For this review, use the dimensioned drawing (mm, ordinates from the lowest corner) and the shaded views. A direction names the side the tool comes from. Coordinates: 2 decimals unless noted, no trailing zeros. Write each loop counter-clockwise with the first axis right and the second up, starting at its lowest first coordinate (ties: lowest second). Pieces come first, ordered by that corner, then holes. Notation, with made-up numbers: (37, 82) - (66, 82) arc R8 ccw to (66, 94) - close; hole circle Ø6 at (33.5, -28.5). An arc over 180 degrees is marked (long way). Put each result on its own line as item: value.
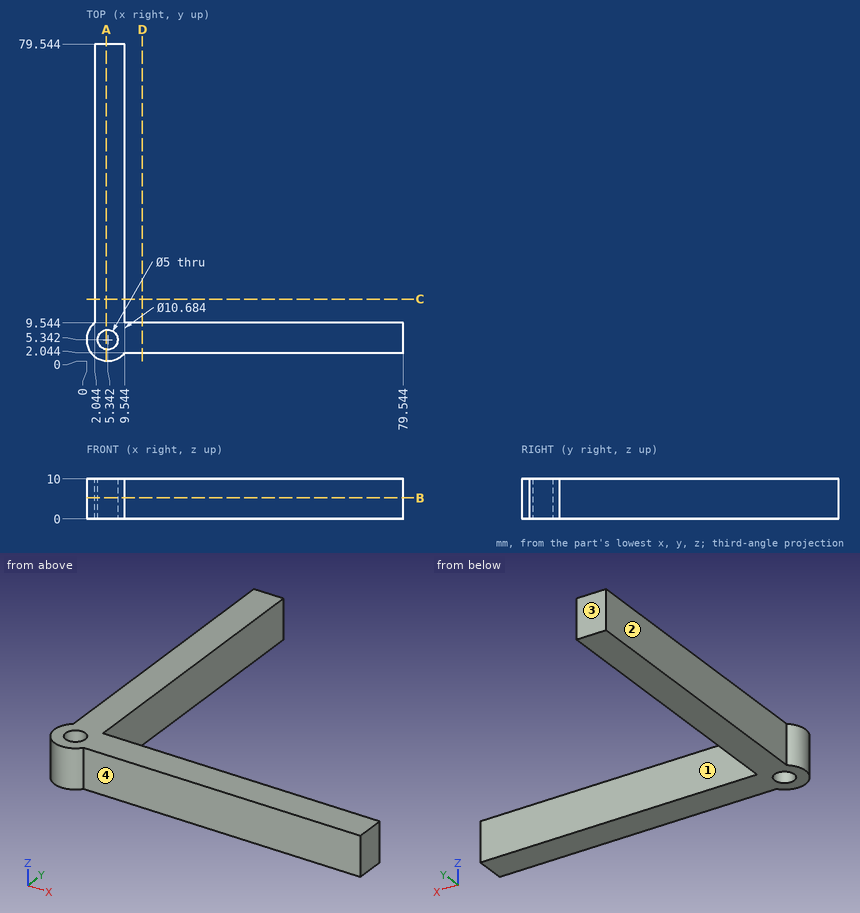
1. Consider section B-B on z = 5.25. State the section outline as (x, y) points (1 decimal), plus the area to 3 significant figures.
Determined:
outline: (2, 9.5) arc R5.3 ccw (long way) to (9.5, 2) - (79.5, 2) - (79.5, 9.5) - (9.5, 9.5) - (9.5, 79.5) - (2, 79.5) - close; hole circle Ø5 at (5.3, 5.3)
area: 1,110 mm^2
2. Machinability: for the marked faces 1, 2, 3 and 4, which of the approach directions +Z, -Z, +X, -X, +Y, -Y give a long, thin tool a straight path to every point of the face, cutting with its end or side? Answer none if there is none.
Determined:
face 1: +Z, -Z, +X, +Y
face 2: +Z, -Z, -X, +Y
face 3: +Z, -Z, +X, -X, +Y
face 4: +Z, -Z, +X, -Y
3. Consider section C-C on y = 15.5. State the section outline as (x, z) points (1 decimal).
Determined:
outline: (2, 0) - (9.5, 0) - (9.5, 10) - (2, 10) - close
4. To check wall thickness, follow probe 1 along Y at (x, z) = (5, 8.75) (1 decimal); probe 2 along X at (y, z) = (42, 9.5) (1 decimal). State the ranges of each line that lie inside material, in increasing order.
Determined:
probe 1: y = 0 to 2.9, 7.8 to 79.5
probe 2: x = 2 to 9.5
5. For pin 1 Ø1 at (x, z) = (16, 9) entering from -Y; pin 2 Ø6 at (x, y) = (15.5, 60) entering from -Z; pin 3 Ø4 at (y, z) = (48.5, 1) entering from -X, all flat-tipped, find the tip position at first contact; note any pin that passes through.
Determined:
pin 1: stops at y = 2.04
pin 2: passes through
pin 3: stops at x = 2.04
6. Consider section A-A on x = 5. State the section outline as (y, z) points (1 decimal).
Determined:
outline: (0, 0) - (2.9, 0) - (2.9, 10) - (0, 10) - close; (7.8, 0) - (79.5, 0) - (79.5, 10) - (7.8, 10) - close
